The drawing under review shows one solid part. Ordinate dimensions are in mm from its lowest x, y, z. A direction names the side the tool comes from. Round coordinates to 2 decimals unless told otherwise and drop trailing zeros. Write each loop counter-clockwise with the first axis right and the second up, starting at its lowest first coordinate (ties: lowest second). Pieces come first, ordered by that corner, then holes. Notation, with made-up numbers: (17, 89) -> (59, 89) arc R18 ccw to (59, 104) -> close; hole circle Ø9 at (-11.75, 26). An arc over 180 degrees is marked (long way). Answer in a Markdown table with one row per item.
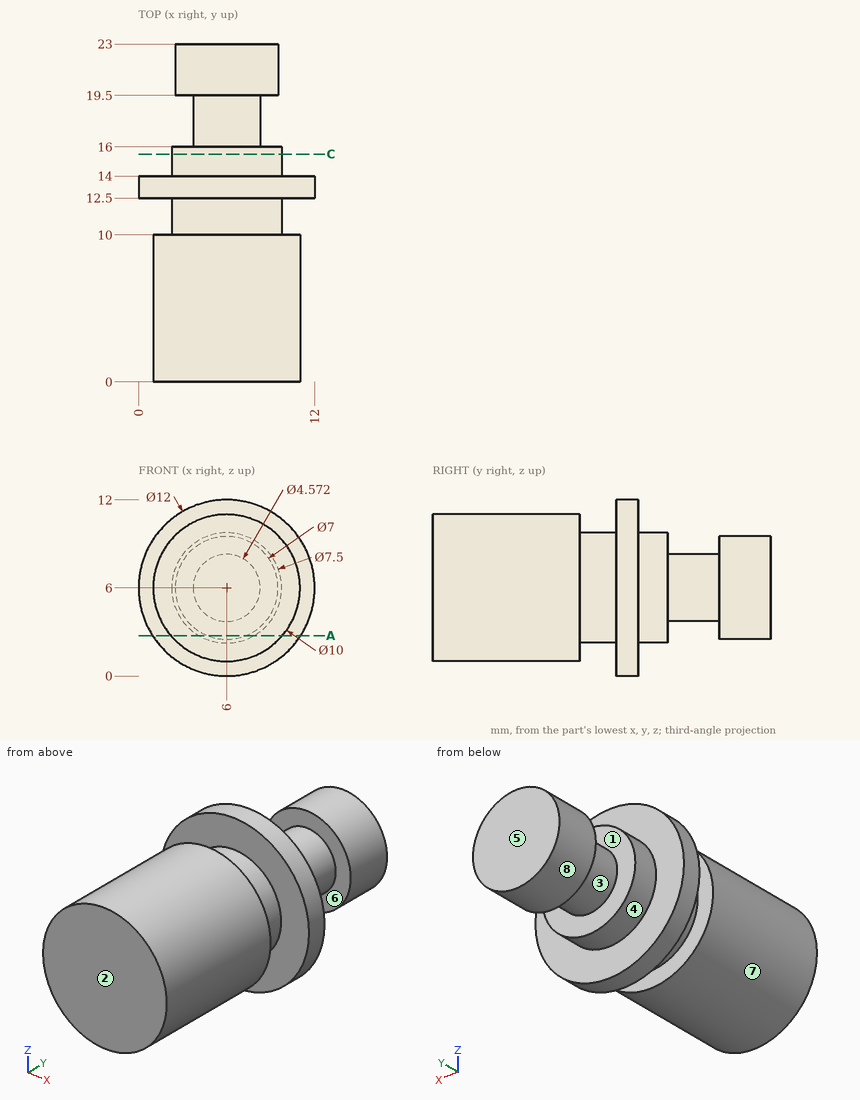
1) Consider section C-C on y = 15.5. State the section outline as (x, z) points, then the cut area to 3 significant figures.
Solved:
| item | result |
|---|---|
| outline | circle Ø7.5 at (6, 6) |
| area | 44.2 mm² |
2) For line 1 (Y direction, x = 4, z = 4.5); line 2 (Y direction, x = 2.25, z = 3); line 3 (Y direction, x = 11.25, z = 7.5), list the stretches that pass through material, from the lowest coordinate up. Write a range as [from, to].
Solved:
| item | result |
|---|---|
| line 1 | [0, 16], [19.5, 23] |
| line 2 | [0, 10], [12.5, 14] |
| line 3 | [12.5, 14] |
3) Clearance check with flat-ended pins moving along their axes: pin 1 Ø6 at (y, z) = (4.5, 7) entering from -X; pin 2 Ø3 at (y, z) = (16.5, 5.5) entering from -X; pin 3 Ø6 at (x, z) = (7, 5.5) entering from -Y; pin 4 Ø6 at (y, z) = (2.5, 3) entering from +X. State where each tip first meets the part, or that it passes through.
Solved:
| item | result |
|---|---|
| pin 1 | x = 1 |
| pin 2 | x = 2.25 |
| pin 3 | y = 0 |
| pin 4 | x = 11 |
4) For the marked faces 5, 6, 7 and 8, list the 3-axis set-ups (+Z, -Z, +X, -X, +Y, -Y) from which the entire face can be reached by the end or side of a thin tool; tool diameter is ignored.
Solved:
| item | result |
|---|---|
| face 5 | +Z, -Z, +X, -X, +Y |
| face 6 | none |
| face 7 | -Y |
| face 8 | +Y |
5) Mouldability with a two-part tool opening along Y and no side actions: class the marked faces 1, 2, 3 and 4 as pulls with the +Y half, pulls with the -Y half, needs draft (parallel to the pull), parting line crosses it, or undercut.
Solved:
| item | result |
|---|---|
| face 1 | undercut |
| face 2 | pulls with the -Y half |
| face 3 | undercut |
| face 4 | needs draft |
6) Consider section A-A on z = 2.75. State the section outline as (x, y) points.
Solved:
| item | result |
|---|---|
| outline | (0.96, 12.5) -> (4.13, 12.5) -> (4.13, 10) -> (2.2, 10) -> (2.2, 0) -> (9.8, 0) -> (9.8, 10) -> (7.87, 10) -> (7.87, 12.5) -> (11.04, 12.5) -> (11.04, 14) -> (7.87, 14) -> (7.87, 16) -> (4.13, 16) -> (4.13, 14) -> (0.96, 14) -> close; (4.7, 19.5) -> (7.3, 19.5) -> (7.3, 23) -> (4.7, 23) -> close |
